Work out the finished part from the listing and answer in its coordinate system (mm). A direction names the side the tool comes from. Round coordinates to 2 decimals unless told otherwise and drop trailing zeros. Order: outer loops, then holes, each group sorted by start corner. A loop starts at its lowest first (then second) coordinate and runs counter-clockwise, first axis right, second up. Notation, with made-up numbers: (-5, -11.75) - (34, -11.75) arc R11 cw to (34, 8.25) - close; hole circle Ø10 at (35, 27.25). An arc over 180 degrees is marked (long way). One line per question, with ' | ' between items. Start each with the question number.
from build123d import *

# Parameters (mm, degrees)
F1_DEPTH = 2
F0_W     = 23.5
F0_H     = 27
F2_DEPTH = 20


with BuildPart() as f1:
    # F0 (on Front) → F1 (new body)
    with BuildSketch(Plane.XZ):
        Polygon((0, 24.5), (-29.5, 13), (-29.5, -13), (0, -24.5), (29.5, -13), (29.5, 13), align=None)
        with BuildLine():
            ThreePointArc((2, -20), (-1.414214, -21.414214), (0, -18))
            ThreePointArc((0, -18), (1.414214, -18.585786), (2, -20))
        make_face(mode=Mode.SUBTRACT)
        Polygon((-17.5, 13.5), (0, 13.5), (23.5, 13.5), (23.5, -13.5), (0, -13.5), (-17.5, -13.5), (-23.5, -7.5), (-23.5, 7.5), align=None, mode=Mode.SUBTRACT)
        with BuildLine():
            ThreePointArc((0, 18), (-1.414214, 21.414214), (2, 20))
            ThreePointArc((2, 20), (1.414214, 18.585786), (0, 18))
        make_face(mode=Mode.SUBTRACT)
    extrude(amount=F1_DEPTH)

    # F0 (on Front) → F2 (join)
    with BuildSketch(Plane.XZ):
        Polygon((0, -13.5), (0, 13.5), (-17.5, 13.5), (-23.5, 7.5), (-23.5, -7.5), (-17.5, -13.5), align=None)
        with Locations((11.75, 0)):
            Rectangle(F0_W, F0_H)
    extrude(amount=F2_DEPTH)


solid = f1.part
1) Section C-C on y = -9.25 is taken. Give the vertices of the cut face in (x, z), and give its area (3 significant figures).
2) Flat-ended cylindrical pins translate along their axes: pin 1 (10 mm diameter, centred on x = -11.5, y = -3.5, fed in from -Z); pin 2 (2 mm diameter, centred on y = -4.5, z = 16.5, fed in from -X); pin 3 (8 mm diameter, centred on y = -8.5, z = 14, fed in from -X); pin 4 (9 mm diameter, centred on y = -7, z = -4.5, fed in from +X). Find the tip coordinate at first contact, or state that the pin passes through.
3) For faces 1 (the flat face through (-20, -11, 11)), 2 (the flat face through (-23.5, -11, 0)), 3 (the flat face through (-21, -11, -10)), 4 (the flat face through (3, -11, -13.5)), determine the directions among +Z, -Z, +X, -X, +Y, -Y from which every point of the face is accessible in a straight line to the end or side of a thin tool.
4) Section A-A on z = -9.5 is taken. Give the vertices of the cut face in (x, y), and give its area (3 significant figures).
5) Straight lines are drawn through the part: line 1 (Z direction, x = 0, y = -1.5); line 2 (Z direction, x = 17.5, y = -5.5); line 3 (X direction, y = -5.25, z = -5). For each, find the intervals that lie inside material, in ascending order.
6) Section D-D on z = -16 is taken. Give the vertices of the cut face in (x, y), and give its area (3 significant figures).
7) Section B-B on x = -11 is taken. Give the vertices of the cut face in (y, z).
Recorded:
1) outline: (-23.5, -7.5) - (-17.5, -13.5) - (23.5, -13.5) - (23.5, 13.5) - (-17.5, 13.5) - (-23.5, 7.5) - close | area: 1,230 mm²
2) pin 1: stops at z = -21.88 | pin 2: passes through | pin 3: stops at x = -21 | pin 4: stops at x = 23.5
3) face 1: +Z, -X, -Y | face 2: +Z, -Z, -X, -Y | face 3: -Z, -X, -Y | face 4: -Z, +X, -X, -Y
4) outline: (-29.5, -2) - (-21.5, -2) - (-21.5, -20) - (23.5, -20) - (23.5, -2) - (29.5, -2) - (29.5, 0) - (-29.5, 0) - close | area: 928 mm²
5) line 1: z = -24.5 to -22, -18 to 18, 22 to 24.5 | line 2: z = -13.5 to 13.5 | line 3: x = -23.5 to 23.5
6) outline: (-21.8, -2) - (21.8, -2) - (21.8, 0) - (-21.8, 0) - close | area: 87.2 mm²
7) outline: (-20, -13.5) - (-2, -13.5) - (-2, -20.21) - (0, -20.21) - (0, 20.21) - (-2, 20.21) - (-2, 13.5) - (-20, 13.5) - close
